```python
from build123d import *

# Parameters (mm, degrees)
SKETCH1_R           = 1.25
BOSS_EXTRUDE1_DEPTH = 8
SKETCH2_R           = 8
BOSS_EXTRUDE2_DEPTH = 4
CHAMFER1_SIZE       = 2


with BuildPart() as part:
    # Sketch1 → Boss-Extrude1 (new body)
    with BuildSketch(Plane(origin=(0, 0, 0), x_dir=(1, 0, 0), z_dir=(0, 1, 0))):
        with BuildLine():
            ThreePointArc((7.4375, -2.946793809), (11, 0), (7.4375, 2.946793809))
            ThreePointArc((7.4375, 2.946793809), (0, 8), (-7.4375, 2.946793809))
            ThreePointArc((-7.4375, 2.946793809), (-11, 0), (-7.4375, -2.946793809))
            ThreePointArc((-7.4375, -2.946793809), (0, -8), (7.4375, -2.946793809))
        make_face()
        with Locations((8, 0)):
            Circle(SKETCH1_R, mode=Mode.SUBTRACT)
        with Locations((-8, 0)):
            Circle(SKETCH1_R, mode=Mode.SUBTRACT)
    extrude(amount=BOSS_EXTRUDE1_DEPTH)

    # Sketch2 → Boss-Extrude2 (add)
    with BuildSketch(Plane(origin=(0, 8, 0), x_dir=(1, 0, 0), z_dir=(0, 1, 0))):
        Circle(SKETCH2_R)
    extrude(amount=BOSS_EXTRUDE2_DEPTH)

    # Chamfer1
    chamfer1_edges = [part.edges().sort_by_distance(p)[0] for p in [
        (-8, 12, 0),
    ]]
    chamfer(chamfer1_edges, length=CHAMFER1_SIZE)

    # Sketch3 → Revolve2 (revolve)
    with BuildSketch(Plane.XY):
        with BuildLine():
            Line((0, 15), (0, 3))
            ThreePointArc((0, 3), (6, 9), (0, 15))
        make_face()
    revolve(axis=Axis((0, 12, 0), (0, -1, 0)))


solid = part.part
```
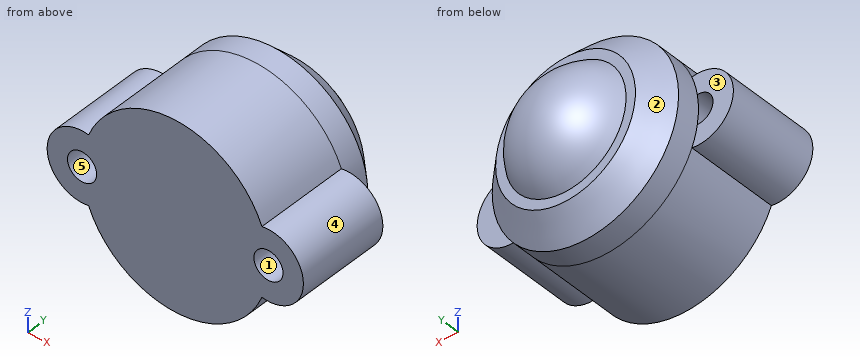
Work out the finished part from the listing and answer in its coordinate system (mm). Face numbers are marked on the shaded views. A direction names the side the tool comes from. Round coordinates to 2 decimals unless told otherwise and drop trailing zeros. Write each loop counter-clockwise with the first axis right and the second up, starting at its lowest first coordinate (ties: lowest second). Pieces come first, ordered by that corner, then holes. Notation, with made-up numbers: (-20, 5) -> (31, 5) arc R20 ccw to (31, 42) -> close; hole circle Ø11 at (-27.75, 40.5). An arc over 180 degrees is marked (long way). Write each question's results on one line, items separated by ' | '.
1) For a pull along Z with two mould halves and no side action, classify the marked faces 3, 4 and 5 as +Z half, -Z half, draft (parallel to the pull), parting line (faces both ways), or undercut.
Findings:
face 3: draft | face 4: parting line | face 5: undercut
2) The part is cut by section C-C (x = -9). Write down the section's boundary in (y, z), and give its area (3 significant figures).
Findings:
outline: (0, -2.83) -> (8, -2.83) -> (8, -0.75) -> (0, -0.75) -> close; (0, 0.75) -> (8, 0.75) -> (8, 2.83) -> (0, 2.83) -> close | area: 33.3 mm²
3) Flat-ended cylindrical pins translate along their axes: pin 1 (4 mm diameter, centred on x = -4.5, y = 10, fed in from +Z); pin 2 (0.6 mm diameter, centred on x = -7.5, z = -0.5, fed in from -Y); pin 3 (4 mm diameter, centred on x = -6.5, z = -2, fed in from +Y). Find the tip coordinate at first contact, or state that the pin passes through.
Findings:
pin 1: stops at z = 7.6 | pin 2: stops at y = 8 | pin 3: stops at y = 12.6
4) Which of the six approach directions +Z, -Z, +X, -X, +Y, -Y give full straight-line access (tool end or side, diameter ignored) to the marked faces 1 and 2?
Findings:
face 1: -Y | face 2: +Y
5) The part is cut by section A-A (z = 0). Write down the section's boundary in (x, y).
Findings:
outline: (-11, 0) -> (-9.25, 0) -> (-9.25, 8) -> (-11, 8) -> close; (-8, 8) -> (-6.75, 8) -> (-6.75, 0) -> (6.75, 0) -> (6.75, 8) -> (8, 8) -> (8, 10) -> (6, 12) -> (5.2, 12) arc R6 ccw to (-5.2, 12) -> (-6, 12) -> (-8, 10) -> close; (9.25, 0) -> (11, 0) -> (11, 8) -> (9.25, 8) -> close
6) The part is cut by section B-B (y = 1.25). Write down the section's boundary in (x, z), and give its area (3 significant figures).
Findings:
outline: (-7.44, -2.95) arc R8 ccw to (7.44, -2.95) arc R3 ccw (long way) to (7.44, 2.95) arc R8 ccw to (-7.44, 2.95) arc R3 ccw (long way) to start; hole circle Ø2.5 at (-8, 0); hole circle Ø2.5 at (8, 0) | area: 222 mm²
7) The part is cut by section D-D (x = 0). Write down the section's boundary in (y, z).
Findings:
outline: (0, -8) -> (10, -8) -> (12, -6) -> (12, -5.2) arc R6 ccw to (12, 5.2) -> (12, 6) -> (10, 8) -> (0, 8) -> close
8) Consider line 1 along Z through (x, y) = (8, 2.5); line 2 along Y through (x, z) = (-8, 2.5); line 3 along X through (y, z) = (9.25, -0.25). Determine where each line is inside the solid, lowest interval first. Write a range as [from, to].
Findings:
line 1: z = [-3, -1.25], [1.25, 3] | line 2: y = [0, 8] | line 3: x = [-8, 8]
